Geometry check sheet. Reference: the model listing, model coordinates, mm. Face numbers are marked on the shaded views. A direction names the side the tool comes from. Round coordinates to 2 decimals unless told otherwise and drop trailing zeros. Order: outer loops, then holes, each group sorted by start corner. A loop starts at its lowest first (then second) coordinate and runs counter-clockwise, first axis right, second up. Notation, with made-up numbers: (-39.75, 89.5) - (-32.75, 89.5) arc R11 cw to (-32.75, 95.5) - close; hole circle Ø6 at (-35, -11.75). An arc over 180 degrees is marked (long way). One line per question, with ' | ' between items. Start each with the question number.
Q1. Sectioned sample at D-D, the plane z = 14.5. Enter the section's corners in (x, y), then the cut area to 3 significant figures.
Q2. Mould release check, pull along Y, two halves, no side actions. Record for the marked faces 1, 2 and 3: +Y half, -Y half, draft (parallel to the pull), parting line (faces both ways), or undercut.
Q3. Sectioned sample at C-C, the plane x = 0. Enter the section's corners in (y, z), then the cut area to 3 significant figures.
Q4. Material ranges on line 1 along X through (y, z) = (-20.85, 42); line 2 along Z through (x, y) = (3.5, -12.5); line 3 along Y through (x, z) = (-1.5, 5.5), recorded low to high.
Q5. Sectioned sample at B-B, the plane z = 42. Enter the section's corners in (x, y), then the cut area to 3 significant figures.
Q6. Tool access check on the marked faces 4, 5, 6, 7 and 8. Record the directions out of +Z, -Z, +X, -X, +Y, -Y that give a thin tool (end or side, any length) a straight path to the whole face; none if there is none.
Q7. Gauge pin test, flat ends, axial feed: P1, Ø3.5, axis at x = -0.5, z = 95, coming from the +Y side; P2, Ø12, axis at y = -2, z = 73, coming from the +X side; P3, Ø6.5, axis at x = -19.5, z = 42, coming from the +Y side. Record the tip position at first contact, or that the pin passes through.
Q8. Sectioned sample at A-A, the plane x = -19.5. Enter the section's corners in (y, z), then the cut area to 3 significant figures.
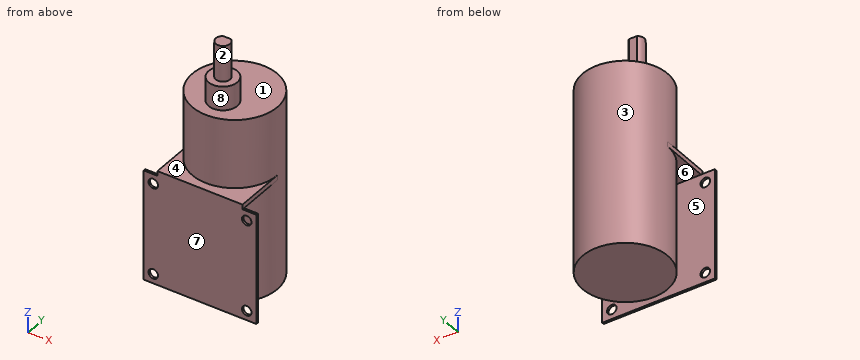
```python
from build123d import *

# Parameters (mm, degrees)
SKETCH1_R           = 17.75
BOSS_EXTRUDE1_DEPTH = 46
BOSS_EXTRUDE2_DEPTH = 2
BOSS_EXTRUDE3_DEPTH = 46
SKETCH4_R           = 17.75
BOSS_EXTRUDE4_DEPTH = 28.7
SKETCH5_R           = 6
BOSS_EXTRUDE5_DEPTH = 10
SKETCH6_R           = 3
BOSS_EXTRUDE6_DEPTH = 15
CUT_EXTRUDE1_START  = -12
CUT_EXTRUDE1_DEPTH  = 12
SKETCH8_R           = 2
CUT_EXTRUDE7_DEPTH  = 12


with BuildPart() as part:
    # Sketch1 → Boss-Extrude1 (new body)
    with BuildSketch(Plane.XY):
        Circle(SKETCH1_R)
    extrude(amount=BOSS_EXTRUDE1_DEPTH)

    # Sketch2 → Boss-Extrude2 (add)
    with BuildSketch(Plane.XY.offset(46)):
        with BuildLine():
            Line((-17.75, -21.25), (17.75, -21.25))
            Line((17.75, -21.25), (17.75, 0))
            ThreePointArc((17.75, 0), (0, 17.75), (-17.75, 0))
            Line((-17.75, 0), (-17.75, -21.25))
        make_face()
    extrude(amount=BOSS_EXTRUDE2_DEPTH)

    # Sketch3 → Boss-Extrude3 (add)
    with BuildSketch(Plane(origin=(0, 0, 46), x_dir=(-1, 0, 0), z_dir=(0, 0, -1))):
        Polygon((0, -21.25), (23.5, -21.25), (23.5, -20.35), (-23.5, -20.35), (-23.5, -21.25), align=None)
    extrude(amount=BOSS_EXTRUDE3_DEPTH)

    # Sketch4 → Boss-Extrude4 (add)
    with BuildSketch(Plane.XY.offset(48)):
        Circle(SKETCH4_R)
    extrude(amount=BOSS_EXTRUDE4_DEPTH)

    # Sketch5 → Boss-Extrude5 (add)
    with BuildSketch(Plane.XY.offset(76.7)):
        with Locations((0, -7.25)):
            Circle(SKETCH5_R)
    extrude(amount=BOSS_EXTRUDE5_DEPTH)

    # Sketch6 → Boss-Extrude6 (add)
    with BuildSketch(Plane.XY.offset(86.7)):
        with Locations((0, -7.25)):
            Circle(SKETCH6_R)
    extrude(amount=BOSS_EXTRUDE6_DEPTH)

    # Sketch7 → Cut-Extrude1 (cut)
    with BuildSketch(Plane.XY.offset(101.7).offset(CUT_EXTRUDE1_START)):
        with BuildLine():
            Line((-1.658312395, -4.75), (1.658312395, -4.75))
            ThreePointArc((1.658312395, -4.75), (0, -4.25), (-1.658312395, -4.75))
        make_face()
    extrude(amount=CUT_EXTRUDE1_DEPTH, mode=Mode.SUBTRACT)

    # Sketch8 → Cut-Extrude7 (cut)
    with BuildSketch(Plane(origin=(0, -21.25, 0), x_dir=(-1, 0, 0), z_dir=(0, -1, 0))):
        with Locations(Location((19.5, -42, 0), (0, 0, 90))):
            Circle(SKETCH8_R)
        with Locations(Location((-19.5, -42, 0), (0, 0, 90))):
            Circle(SKETCH8_R)
        with Locations(Location((19.5, -4, 0), (0, 0, 90))):
            Circle(SKETCH8_R)
        with Locations(Location((-19.5, -4, 0), (0, 0, 90))):
            Circle(SKETCH8_R)
    extrude(amount=-CUT_EXTRUDE7_DEPTH, mode=Mode.SUBTRACT)


solid = part.part
```
Determined:
1) outline: (-23.5, -21.25) - (23.5, -21.25) - (23.5, -20.35) - (-23.5, -20.35) - close; circle Ø35.5 at (0, 0) | area: 1,030 mm2
2) face 1: draft | face 2: parting line | face 3: undercut
3) outline: (-21.25, 0) - (-20.35, 0) - (-20.35, 46) - (-17.75, 46) - (-17.75, 0) - (17.75, 0) - (17.75, 76.7) - (-1.25, 76.7) - (-1.25, 86.7) - (-4.25, 86.7) - (-4.25, 89.7) - (-4.75, 89.7) - (-4.75, 101.7) - (-10.25, 101.7) - (-10.25, 86.7) - (-13.25, 86.7) - (-13.25, 76.7) - (-17.75, 76.7) - (-17.75, 48) - (-21.25, 48) - close | area: 2,980 mm2
4) line 1: x = -23.5 to -21.5, -17.5 to 17.5, 21.5 to 23.5 | line 2: z = 0 to 76.7 | line 3: y = -21.25 to -20.35, -17.69 to 17.69
5) outline: (-23.5, -21.25) - (-21.5, -21.25) - (-21.5, -20.35) - (-23.5, -20.35) - close; circle Ø35.5 at (0, 0); (-17.5, -21.25) - (17.5, -21.25) - (17.5, -20.35) - (-17.5, -20.35) - close; (21.5, -21.25) - (23.5, -21.25) - (23.5, -20.35) - (21.5, -20.35) - close | area: 1,020 mm2
6) face 4: +Z, -Y | face 5: -Z, +X, -X | face 6: -Z | face 7: +Z, -Z, +X, -X, -Y | face 8: +Z
7) P1: stops at y = -4.75 | P2: stops at x = 17.75 | P3: stops at y = 7.14
8) outline: (-21.25, 0) - (-20.35, 0) - (-20.35, 2) - (-21.25, 2) - close; (-21.25, 6) - (-20.35, 6) - (-20.35, 40) - (-21.25, 40) - close; (-21.25, 44) - (-20.35, 44) - (-20.35, 46) - (-21.25, 46) - close | area: 34.2 mm2
